Autodesk Inventor part; units mm, degrees
ref_plane "YZ Plane" through (0, 0, 0) normal (1, 0, 0) x (0, 1, 0)
ref_plane "XZ Plane" through (0, 0, 0) normal (0, 1, 0) x (-1, 0, 0)
ref_plane "XY Plane" through (0, 0, 0) normal (0, 0, 1) x (1, 0, 0)
sketch "Sketch1" plane through (0, 0, 0) normal (1, 0, 0) x (0, 1, 0)
  line L0 (25, 22.5) -> (-25, 22.5)
  line L1 (-25, 22.5) -> (-25, -100)
  line L2 (-25, -100) -> (25, -100)
  line L3 (25, -100) -> (25, 22.5)
  circle A0 centre (0, 0) radius 25
  circle A1 centre (0, 0) radius 20
  circle A2 centre (0, 0) radius 3.2936
  point P0 (25, 0)
  point P1 (-25, 0)
  dimension "d0" = 50
  dimension "d1" = 122.5
  dimension "d2" = 25
  dimension "d3" = 22.5
  dimension "d12" = 40
  dimension "d13" = 6.5872
extrude "Extrusion1" add sketch "Sketch1" along normal blind 5 contours A0 L0 | L0 A0 | L3 L2 L1 A0 | A1
sketch "Sketch4" plane through (5, 0, 0) normal (1, 0, 0) x (0, 0, -1)
  line L0 (100, -25) -> (100, 25)
  line L1 (100, 25) -> (0, 25)
  line L2 (100, -25) -> (0, -25)
  line L3 (0, -25) -> (0, 25)
  line L4 (0, 25) -> (100, 25)
  line L5 (100, 25) -> (100, -25)
  circle A0 centre (0, 0) radius 3.2936
  arc A1 (15, 20) -> (15, -20) centre (0, 0) ccw
  circle A2 centre (0, 0) radius 20
  line L6 (0, 20) -> (95, 20)
  line L7 (95, 20) -> (95, -20)
  line L8 (95, -20) -> (0, -20)
  line L9 (0, -20) -> (0, 20)
  point P0 (0, -20)
  dimension "d15" = 40
  dimension "d14" = 50
  dimension "d16" = 5
  dimension "d17" = 5
extrude "Extrusion3" add sketch "Sketch4" along normal blind 45 contours L2 A1 L8 L7 L6 L1 L0 | A1 L3 A2 | L3 L8 A1 | A1 L6 L3
sketch "Sketch5" plane through (50, 0, 0) normal (1, 0, 0) x (0, 0, -1)
  line L0 (100, -25) -> (100, 25)
  line L1 (0, 25) -> (100, 25)
  line L2 (100, 25) -> (100, -25)
  line L3 (100, -25) -> (0, -25)
  line L4 (0, -25) -> (0, 25)
  circle A0 centre (0, 0) radius 25
  arc A1 (0, 20) -> (0, -20) centre (0, 0) ccw
  circle A2 centre (0, 0) radius 15
  line L5 (0, 15) -> (35, 15)
  line L6 (35, 15) -> (35, -15)
  line L7 (35, -15) -> (0, -15)
  line L8 (0, -15) -> (0, 15)
  point P0 (0, -15)
  point P1 (100, 25)
  dimension "d20" = 30
  dimension "d21" = 10
  dimension "d22" = 50
  dimension "d23" = 35
extrude "Extrusion4" add sketch "Sketch5" against normal blind 5 contours L3 A0 L7 L6 L5 L1 L0 | A0 L4 A1 | L4 L7 A0 | A0 L5 L4 | A1 L4 A2
sketch "Sketch6" plane through (5, 0, 0) normal (1, 0, 0) x (0, 0, -1)
  circle A0 centre (0, 0) radius 20
  line L0 (95, 20) -> (0, 20)
  line L1 (0, -20) -> (95, -20)
  line L2 (0, 20) -> (22, 20)
  line L3 (22, 20) -> (22, -20)
  line L4 (22, -20) -> (0, -20)
  line L5 (0, -20) -> (0, 20)
  dimension "d26" = 22
extrude "Extrusion5" add sketch "Sketch6" along normal blind 20
sketch "Sketch7" plane through (0, 0, 0) normal (-1, 0, 0) x (0, 0, 1)
  circle A0 centre (0, 0) radius 9.5
  dimension "d29" = 19
extrude "Extrusion6" cut sketch "Sketch7" against normal blind 12.5
sketch "Sketch8" plane through (0, 0, 0) normal (-1, 0, 0) x (0, 0, 1)
  circle A0 centre (0, 0) radius 11.5
  dimension "d32" = 23
extrude "Extrusion7" cut sketch "Sketch8" against normal blind 6.5
sketch "Sketch9" plane through (12.5, 0, 0) normal (-1, 0, 0) x (0, 0, 1)
  circle A0 centre (0, 0) radius 9.5
  circle A1 centre (0, 0) radius 6.2
  line L0 (0, 0) -> (7.2952, 0)
  line L1 (0, 0) -> (-3.8354, 6.643)
  line L2 (0, 0) -> (-3.5239, -6.1036)
  circle A2 centre (-3.1, 5.3694) radius 1.45
  circle A3 centre (6.2, 0) radius 1.45
  circle A4 centre (-3.1, -5.3694) radius 1.45
  dimension "d35" = 12.4
  dimension "d36" = 120
  dimension "d37" = 120
  dimension "d38" = 2.9
  dimension "d39" = 2.9
  dimension "d40" = 2.9
extrude "Extrusion8" cut sketch "Sketch9" against normal blind 16 contours L0 A3 A1 | A1 A3 | A1 A3 L0 | A2 L1 A1 | A1 L1 A2 | A4 A1 | A1 L2 A4 | L1 A2 A1 | A1 A2 L1 | A1 A4 L2
sketch "Sketch10" plane through (25, 0, 0) normal (1, 0, 0) x (0, 0, -1)
  circle A0 centre (3.1, 5.3694) radius 1.45
  circle A1 centre (3.1, 5.3694) radius 4
  circle A2 centre (3.1, -5.3694) radius 1.45
  circle A3 centre (3.1, -5.3694) radius 4
  circle A4 centre (-6.2, 0) radius 1.45
  circle A5 centre (-6.2, 0) radius 4
  point P0 (0, 0)
  dimension "d43" = 8
  dimension "d44" = 8
  dimension "d45" = 8
extrude "Extrusion9" cut sketch "Sketch10" against normal blind 7
sketch "Sketch11" plane through (0, 25, 0) normal (0, 1, 0) x (1, 0, 0)
  line L0 (0, 100) -> (50, 100)
  line L1 (0, 100) -> (0, 0)
  line L2 (50, 100) -> (0, 100)
  line L3 (0, 100) -> (0, 45)
  line L4 (0, 45) -> (50, 45)
  line L5 (50, 45) -> (50, 100)
  line L6 (50, 0) -> (50, 100)
  line L7 (50, 100) -> (25, 100)
  line L8 (25, 100) -> (25, 45)
  line L9 (25, 45) -> (50, 45)
  line L10 (50, 45) -> (50, 100)
  dimension "d48" = 55
extrude "Extrusion10" cut sketch "Sketch11" against normal blind 50 contours L0 L5 L4 L8
sketch "Sketch12" plane through (5, 0, 0) normal (1, 0, 0) x (0, 0, -1)
  line L0 (95, 20) -> (22, 20)
  line L1 (22, -20) -> (95, -20)
  line L2 (95, 20) -> (45, 20)
  line L3 (45, 20) -> (45, -20)
  line L4 (45, -20) -> (95, -20)
  line L5 (95, -20) -> (95, 20)
  point P0 (0, 0)
  dimension "d51" = 50
extrude "Extrusion11" add sketch "Sketch12" along normal blind 20
sketch "Sketch13" plane through (25, 25, -45) normal (1, 0, 0) x (0, 0, -1)
  line L0 (10, -10) -> (45, -10)
  line L1 (45, -10) -> (45, -40)
  line L2 (45, -40) -> (10, -40)
  line L3 (10, -40) -> (10, -10)
  line L4 (0, 0) -> (55, 0)
  line L5 (55, 0) -> (55, -50)
  line L6 (55, -50) -> (0, -50)
  line L7 (0, -50) -> (0, 0)
  circle A0 centre (10, -10) radius 1.95
  circle A1 centre (10, -40) radius 1.95
  circle A2 centre (45, -40) radius 1.95
  circle A3 centre (45, -10) radius 1.95
  point P0 (-45, -25)
  dimension "d54" = 10
  dimension "d55" = 10
  dimension "d56" = 10
  dimension "d57" = 10
  dimension "d58" = 3.9
  dimension "d59" = 3.9
  dimension "d60" = 3.9
  dimension "d61" = 3.9
extrude "Extrusion12" cut sketch "Sketch13" against normal blind 26 contours L3 A0 L0 | L0 A0 L3 | A3 L1 L0 | L0 L1 A3 | A1 L2 L3 | L3 L2 A1 | A2 L2 L1 | L1 L2 A2
sketch "Sketch14" plane through (0, 0, 0) normal (-1, 0, 0) x (0, 0, 1)
  circle A0 centre (-90, 15) radius 1.95
  circle A1 centre (-90, 15) radius 4
  circle A2 centre (-55, 15) radius 1.95
  circle A3 centre (-55, 15) radius 4
  circle A4 centre (-55, -15) radius 1.95
  circle A5 centre (-55, -15) radius 4
  circle A6 centre (-90, -15) radius 1.95
  circle A7 centre (-90, -15) radius 4
  point P0 (0, 0)
  dimension "d64" = 8
  dimension "d65" = 8
  dimension "d66" = 8
  dimension "d67" = 8
extrude "Extrusion13" cut sketch "Sketch14" against normal blind 10 contours A0 | A1 | A2 | A3 | A5 | A7
sketch "Sketch15" plane through (5, 0, 0) normal (1, 0, 0) x (0, 0, -1)
  line L0 (45, -20) -> (45, 20)
  line L1 (22, -20) -> (45, -20)
  line L2 (45, 20) -> (22, 20)
  line L3 (22, 20) -> (22, -20)
  line L4 (22, -20) -> (45, -20)
  line L5 (45, -20) -> (45, 20)
  point P0 (0, 0)
extrude "Extrusion14" add sketch "Sketch15" along normal blind 20
properties part number "Link2_v2a"
For this review, take the finished solid that the model builds, in its own axes (mm). A direction names the side the tool comes from. Coordinates: 2 decimals unless noted, no trailing zeros. Write each loop counter-clockwise with the first axis right and the second up, starting at its lowest first coordinate (ties: lowest second). Pieces come first, ordered by that corner, then holes. Notation, with made-up numbers: (-24.75, 43.5) -> (7.25, 43.5) arc R14 ccw to (7.25, 51.5) -> close; hole circle Ø5 at (50, 20.25). An arc over 180 degrees is marked (long way). Put each result on its own line as item: value.
Q1. Clearance check with flat-ended pins moving along their axes: pin 1 Ø4 at (y, z) = (-5.37, -3.1) entering from +X; pin 2 Ø12 at (x, y) = (35, -16) entering from -Z; pin 3 Ø4 at (y, z) = (-4, -5) entering from +X; pin 4 Ø5 at (x, z) = (29, -70) entering from -Y. State where each tip first meets the part, or that it passes through.
From the geometry:
pin 1: stops at x = 18
pin 2: stops at z = -45
pin 3: stops at x = 25
pin 4: passes through
Q2. Take a section at A-A, the plane z = -55. State the section outline as (x, y) points, then the cut area to 3 significant figures.
From the geometry:
outline: (0, -25) -> (25, -25) -> (25, -16.95) -> (10, -16.95) -> (10, -19) -> (0, -19) -> close; (0, -11) -> (10, -11) -> (10, -13.05) -> (25, -13.05) -> (25, 13.05) -> (10, 13.05) -> (10, 11) -> (0, 11) -> close; (0, 19) -> (10, 19) -> (10, 16.95) -> (25, 16.95) -> (25, 25) -> (0, 25) -> close
area: 973 mm2
Q3. Wall thickness on L1, parallel to Y at x = 6.5, z = -90; L2, parallel to Y at x = 16, z = -55; L3, parallel to X at y = 17, z = -25: over which ranges is each line inside the solid? List them lowest first.
From the geometry:
L1: y = -25 to -19, -11 to 11, 19 to 25
L2: y = -25 to -16.95, -13.05 to 13.05, 16.95 to 25
L3: x = 0 to 25, 45 to 50
Q4. Tool access review of faces 1 (the cylindrical face through (4.93, 17.7, -92.95)), 2 (the flat face through (48, 15, -17)), 3 (the flat face through (45, -16, -17)): name each direction out of +Z, -Z, +X, -X, +Y, -Y from which nothing blocks a thin tool from reaching the whole face with its end or side.
From the geometry:
face 1: -X
face 2: +X
face 3: -Z
Q5. Take a section at B-B, the plane x = 39.5. State the section outline as (y, z) points.
From the geometry:
outline: (-25, -45) -> (-20, -45) -> (-20, 0) arc R20 cw to (20, 0) -> (20, -45) -> (25, -45) -> (25, 0) arc R25 ccw to (-25, 0) -> close
Q6. Take a section at D-D, the plane x = 22.5. State the section outline as (y, z) points.
From the geometry:
outline: (-25, -100) -> (25, -100) -> (25, 0) arc R25 ccw to (-25, 0) -> close; hole circle Ø3.9 at (-15, -90); hole circle Ø3.9 at (-15, -55); hole circle Ø8 at (-5.37, -3.1); hole circle Ø8 at (0, 6.2); hole circle Ø8 at (5.37, -3.1); hole circle Ø3.9 at (15, -90); hole circle Ø3.9 at (15, -55)
Q7. The part is to be moulded in two halves that separate along Z. For faces 4 (the flat face through (19, 25, -40)), 5 (the cylindrical face through (35, 0, 20)), 6 (the flat face through (18, 5, -5)), 7 (the cylindrical face through (4.93, -13.799, -51.185)), say which applies: +Z half, -Z half, draft (parallel to the pull), parting line (faces both ways), or undercut.
From the geometry:
face 4: draft
face 5: -Z half
face 6: undercut
face 7: undercut
Q8. Take a section at C-C, the plane z = 6.2. State the section outline as (x, y) points, then the cut area to 3 significant figures.
From the geometry:
outline: (0, -24.22) -> (50, -24.22) -> (50, -13.66) -> (45, -13.66) -> (45, -19.01) -> (25, -19.01) -> (25, -4) -> (18, -4) -> (18, -1.45) -> (12.5, -1.45) -> (12.5, -7.2) -> (6.5, -7.2) -> (6.5, -9.69) -> (0, -9.69) -> close; (0, 9.69) -> (6.5, 9.69) -> (6.5, 7.2) -> (12.5, 7.2) -> (12.5, 1.45) -> (18, 1.45) -> (18, 4) -> (25, 4) -> (25, 19.01) -> (45, 19.01) -> (45, 13.66) -> (50, 13.66) -> (50, 24.22) -> (0, 24.22) -> close
area: 1,240 mm2
